Here's how the part is built. I have some questions about the finished solid (model axes, mm). A direction names the side the tool comes from. Round coordinates to 2 decimals unless told otherwise and drop trailing zeros. Write each loop counter-clockwise with the first axis right and the second up, starting at its lowest first coordinate (ties: lowest second). Pieces come first, ordered by that corner, then holes. Notation, with made-up numbers: (36, 26) -> (64, 26) arc R26 cw to (64, 47) -> close; hole circle Ø5 at (78.25, -35.75). An arc over 180 degrees is marked (long way). Answer in a Markdown table with one row per item.
from build123d import *

# Parameters (mm, degrees)
AUFSATZ_LINEAR_AUSTRAGEN1_DEPTH = 180
AUFSATZ_LINEAR_START            = -10
SKIZZE3_W                       = 2
SKIZZE3_H                       = 15
AUFSATZ_LINEAR_AUSTRAGEN2_DEPTH = 10
SKIZZE11_W                      = 12
SKIZZE11_H                      = 15
AUFSATZ_LINEAR_AUSTRAGEN6_DEPTH = 10
SCHNITT_LINEAR_AUSTRAGEN3_DEPTH = 180
AUFSATZ_LINEAR_AUSTRAGEN3_DEPTH = 3
SKIZZE9_W                       = 17.608625436
SKIZZE9_H                       = 6.338284118
AUFSATZ_LINEAR_AUSTRAGEN5_DEPTH = 7
SKIZZE10_R                      = 0.75
SKIZZE10_R_2                    = 1.25
SCHNITT_LINEAR_AUSTRAGEN5_DEPTH = 7
AUFSATZ_LINEAR_AUSTRAGEN7_DEPTH = 3
SKIZZE13_W                      = 7
SKIZZE13_H                      = 7
AUFSATZ_LINEAR_AUSTRAGEN8_DEPTH = 5
SKIZZE15_R                      = 1.75
SCHNITT_LINEAR_AUSTRAGEN6_DEPTH = 5


# Read off the part's stored shape, not the designer's step: Schnitt-Linear austragen3, Aufsatz-Linear austragen3, Aufsatz-Linear austragen7
with BuildPart() as part:
    # Skizze2 → Aufsatz-Linear austragen1 (new body)
    with BuildSketch(Plane(origin=(0, 0, 0), x_dir=(0, 0, -1), z_dir=(1, 0, 0))):
        with BuildLine():
            ThreePointArc((-6.804312718, 5.759216901), (-4.554982705, 7.051387337), (-2, 7.5))
            Line((-2, 7.5), (2, 7.5))
            ThreePointArc((2, 7.5), (9.5, 0), (2, -7.5))
            Line((2, -7.5), (-2, -7.5))
            ThreePointArc((-2, -7.5), (-4.554982705, -7.051387337), (-6.804312718, -5.759216901))
            Line((-6.804312718, -5.759216901), (-6.804312718, -8.195643923))
            ThreePointArc((-6.804312718, -8.195643923), (-4.489114575, -9.16811369), (-2, -9.5))
            Line((-2, -9.5), (2, -9.5))
            ThreePointArc((2, -9.5), (11.5, 0), (2, 9.5))
            Line((2, 9.5), (-2, 9.5))
            ThreePointArc((-2, 9.5), (-4.489114575, 9.16811369), (-6.804312718, 8.195643923))
            Line((-6.804312718, 8.195643923), (-6.804312718, 5.759216901))
        make_face()
    extrude(amount=AUFSATZ_LINEAR_AUSTRAGEN1_DEPTH)

    # Skizze3 → Aufsatz-Linear austragen2 (add)
    with BuildSketch(Plane.XY.offset(AUFSATZ_LINEAR_START)):
        with Locations((37, 0)):
            Rectangle(SKIZZE3_W, SKIZZE3_H)
        with Locations((7, 0)):
            Rectangle(SKIZZE3_W, SKIZZE3_H)
        with Locations((23, 0)):
            Rectangle(SKIZZE3_W, SKIZZE3_H)
        with Locations((53, 0)):
            Rectangle(SKIZZE3_W, SKIZZE3_H)
        with Locations((67, 0)):
            Rectangle(SKIZZE3_W, SKIZZE3_H)
        with Locations((83, 0)):
            Rectangle(SKIZZE3_W, SKIZZE3_H)
        with Locations((97, 0)):
            Rectangle(SKIZZE3_W, SKIZZE3_H)
        with Locations((113, 0)):
            Rectangle(SKIZZE3_W, SKIZZE3_H)
        with Locations((127, 0)):
            Rectangle(SKIZZE3_W, SKIZZE3_H)
        with Locations((143, 0)):
            Rectangle(SKIZZE3_W, SKIZZE3_H)
        with Locations((157, 0)):
            Rectangle(SKIZZE3_W, SKIZZE3_H)
        with Locations((173, 0)):
            Rectangle(SKIZZE3_W, SKIZZE3_H)
    extrude(amount=AUFSATZ_LINEAR_AUSTRAGEN2_DEPTH)

    # Skizze11 → Aufsatz-Linear austragen6 (add)
    with BuildSketch(Plane.XY.offset(AUFSATZ_LINEAR_START)):
        with Locations((30, 0)):
            Rectangle(SKIZZE11_W, SKIZZE11_H)
        with Locations((60, 0)):
            Rectangle(SKIZZE11_W, SKIZZE11_H)
        with Locations((90, 0)):
            Rectangle(SKIZZE11_W, SKIZZE11_H)
        with Locations((120, 0)):
            Rectangle(SKIZZE11_W, SKIZZE11_H)
        with Locations((150, 0)):
            Rectangle(SKIZZE11_W, SKIZZE11_H)
    extrude(amount=AUFSATZ_LINEAR_AUSTRAGEN6_DEPTH)

    # Schnitt-Linear austragen3 outline → Schnitt-Linear austragen3 (cut)
    with BuildSketch(Plane(origin=(0, 0, 0), x_dir=(0, 0, -1), z_dir=(1, 0, 0))):
        with BuildLine():
            ThreePointArc((0, -7.228416147), (5.5, 0), (0, 7.228416147))
            Line((0, 7.228416147), (0, -7.228416147))
        make_face()
        with BuildLine():
            Line((-6.804312718, 8.195643923), (-6.804312718, 8.167645701))
            ThreePointArc((-6.804312718, 8.167645701), (-4.489620266, 9.142956192), (-2, 9.47585653))
            Line((-2, 9.47585653), (2, 9.47585653))
            ThreePointArc((2, 9.47585653), (11.47585653, 0), (2, -9.47585653))
            Line((2, -9.47585653), (-2, -9.47585653))
            ThreePointArc((-2, -9.47585653), (-4.489620266, -9.142956192), (-6.804312718, -8.167645701))
            Line((-6.804312718, -8.167645701), (-6.804312718, -8.195643923))
            ThreePointArc((-6.804312718, -8.195643923), (-4.489114575, -9.16811369), (-2, -9.5))
            Line((-2, -9.5), (2, -9.5))
            ThreePointArc((2, -9.5), (5.082207002, -8.986100378), (7.830951895, -7.5))
            Line((7.830951895, -7.5), (10, -7.5))
            Line((10, -7.5), (10, -5.123475383))
            ThreePointArc((10, -5.123475383), (11.5, 0), (10, 5.123475383))
            Line((10, 5.123475383), (10, 7.5))
            Line((10, 7.5), (7.830951895, 7.5))
            ThreePointArc((7.830951895, 7.5), (5.082207002, 8.986100378), (2, 9.5))
            Line((2, 9.5), (-2, 9.5))
            ThreePointArc((-2, 9.5), (-4.489114575, 9.16811369), (-6.804312718, 8.195643923))
        make_face()
    extrude(amount=SCHNITT_LINEAR_AUSTRAGEN3_DEPTH, mode=Mode.SUBTRACT)

    # Aufsatz-Linear austragen3 outline → Aufsatz-Linear austragen3 (add)
    with BuildSketch(Plane(origin=(180, 0, 0), x_dir=(0, 0, -1), z_dir=(1, 0, 0))):
        with BuildLine():
            Line((-6.804312718, 8.167645701), (-6.804312718, -8.167645701))
            ThreePointArc((-6.804312718, -8.167645701), (-4.489620266, -9.142956192), (-2, -9.47585653))
            Line((-2, -9.47585653), (2, -9.47585653))
            ThreePointArc((2, -9.47585653), (11.47585653, 0), (2, 9.47585653))
            Line((2, 9.47585653), (-2, 9.47585653))
            ThreePointArc((-2, 9.47585653), (-4.489620266, 9.142956192), (-6.804312718, 8.167645701))
        make_face()
    extrude(amount=AUFSATZ_LINEAR_AUSTRAGEN3_DEPTH)

    # Skizze9 → Aufsatz-Linear austragen5 (add)
    with BuildSketch(Plane(origin=(183, 0, 0), x_dir=(0, 0, -1), z_dir=(1, 0, 0))):
        with Locations((2, 0)):
            Rectangle(SKIZZE9_W, SKIZZE9_H)
    extrude(amount=AUFSATZ_LINEAR_AUSTRAGEN5_DEPTH)

    # Skizze10 → Schnitt-Linear austragen5 (cut)
    with BuildSketch(Plane(origin=(190, 0, 0), x_dir=(0, 0, -1), z_dir=(1, 0, 0))):
        with Locations((-4.75, 0)):
            Circle(SKIZZE10_R)
        with Locations((8.75, 0)):
            Circle(SKIZZE10_R)
        with Locations((2, 0)):
            Circle(SKIZZE10_R_2)
    extrude(amount=-SCHNITT_LINEAR_AUSTRAGEN5_DEPTH, mode=Mode.SUBTRACT)

    # Aufsatz-Linear austragen7 outline → Aufsatz-Linear austragen7 (add)
    with BuildSketch(Plane.ZY):
        with BuildLine():
            Line((6.804312718, -8.167645701), (6.804312718, 8.167645701))
            ThreePointArc((6.804312718, 8.167645701), (4.489620266, 9.142956192), (2, 9.47585653))
            Line((2, 9.47585653), (-2, 9.47585653))
            ThreePointArc((-2, 9.47585653), (-11.47585653, 0), (-2, -9.47585653))
            Line((-2, -9.47585653), (2, -9.47585653))
            ThreePointArc((2, -9.47585653), (4.489620266, -9.142956192), (6.804312718, -8.167645701))
        make_face()
    extrude(amount=AUFSATZ_LINEAR_AUSTRAGEN7_DEPTH)

    # Skizze13 → Aufsatz-Linear austragen8 (add)
    with BuildSketch(Plane.ZY.offset(3)):
        with Locations((-2, 0)):
            Rectangle(SKIZZE13_W, SKIZZE13_H)
    extrude(amount=AUFSATZ_LINEAR_AUSTRAGEN8_DEPTH)

    # Skizze15 → Schnitt-Linear austragen6 (cut)
    with BuildSketch(Plane.ZY.offset(8)):
        with Locations((-2, 0)):
            Circle(SKIZZE15_R)
    extrude(amount=-SCHNITT_LINEAR_AUSTRAGEN6_DEPTH, mode=Mode.SUBTRACT)


solid = part.part
1) I need wall thicknesses on line 1 (X direction, y = -5.75, z = -1.25); line 2 (Y direction, x = 188.25, z = -2); line 3 (X direction, y = 1, z = 5.5). Which ranges of each line are inside material? Lowest first, please. Write a range as [from, to].
Response:
| item | result |
|---|---|
| line 1 | x = [-3, 0], [180, 183] |
| line 2 | y = [-3.17, -1.25], [1.25, 3.17] |
| line 3 | x = [-3, 0], [180, 190] |
2) We'd pull the mould along X, two halves only. Please class faces 6 (the face through (190, 1.5, -1.9)), 7 (the face through (14.9, 0.16, -9.5)), 8 (the face through (91.302, 9.134, 4.524)): +X half, -X half, draft (parallel to the pull), parting line (faces both ways), or undercut.
Response:
| item | result |
|---|---|
| face 6 | +X half |
| face 7 | undercut |
| face 8 | draft |
3) For pin 1 (8 mm diameter, centred on x = 58.5, y = 4.5, fed in from -Z); pin 2 (4 mm diameter, centred on x = -5.5, y = 1, fed in from -Z); pin 3 (1 mm diameter, centred on x = 112.5, y = 7, fed in from -Z), each with a flat end and sliding along its axis, tell me the tip position at first contact or that it passes through.
Response:
| item | result |
|---|---|
| pin 1 | stops at z = -11.46 |
| pin 2 | stops at z = -5.5 |
| pin 3 | stops at z = -8.9 |
4) I want a section at A-A, the plane x = 24.5. List the corners of the cut face in (y, z) for me, and give its area (3 significant figures).
Response:
| item | result |
|---|---|
| outline | (-9.48, -2) arc R9.48 ccw to (9.48, -2) -> (9.48, 2) arc R9.48 ccw to (8.17, 6.8) -> (5.76, 6.8) arc R7.5 cw to (7.5, 2) -> (7.5, 0) -> (7.23, 0) arc R7.5 cw to (-7.23, 0) -> (-7.5, 0) -> (-7.5, 2) arc R7.5 cw to (-5.76, 6.8) -> (-8.17, 6.8) arc R9.48 ccw to (-9.48, 2) -> close |
| area | 148 mm^2 |
5) Which directions (+Z, -Z, +X, -X, +Y, -Y) give clear straight access to the entire face, cutting with the end or side of a thin tool? Please do faces 1 (the face through (52, 0, -6)), 2 (the face through (186, 0, -10.804)), 3 (the face through (186, -3.169, -2)), 4 (the face through (-5, 3.5, -2)), 5 (the face through (186, 3.169, -2)).
Response:
| item | result |
|---|---|
| face 1 | none |
| face 2 | -Z, +X, +Y, -Y |
| face 3 | +Z, -Z, +X, -Y |
| face 4 | +Z, -Z, -X, +Y |
| face 5 | +Z, -Z, +X, +Y |
